Autodesk Inventor part; units mm, degrees
ref_plane "YZ Plane" through (0, 0, 0) normal (1, 0, 0) x (0, 1, 0)
ref_plane "XZ Plane" through (0, 0, 0) normal (0, 1, 0) x (-1, 0, 0)
ref_plane "XY Plane" through (0, 0, 0) normal (0, 0, 1) x (1, 0, 0)
sketch "스케치1" plane through (0, 0, 0) normal (0, 0, 1) x (1, 0, 0)
  line L0 (0, 0) -> (0, 30)
  line L1 (0, 30) -> (1.5, 30)
  line L2 (1.5, 30) -> (1.5, 0)
  line L3 (0, -2) -> (3.5, -2)
  line L4 (3.5, -2) -> (1.5, 0)
  line L5 (0, 0) -> (0, -2)
  dimension "d0" = 30
  dimension "d1" = 7
  dimension "d2" = 3
  dimension "d3" = 45
revolve "회전1" add sketch "스케치1" angle 360 about axis through (0, 0, 0) along (0, 1, 0)
chamfer "모따기1" distance 0.3 angle 45 1 edges at (-1.5, 30, 0)
thread "스레드1"
sketch "스케치2" plane through (0, -2, 0) normal (0, -1, 0) x (1, 0, 0)
  line L0 (-0.5, 2.5) -> (0.5, 2.5)
  line L1 (0.5, 2.5) -> (0.5, -2.5)
  line L2 (0.5, -2.5) -> (-0.5, -2.5)
  line L3 (-0.5, -2.5) -> (-0.5, 2.5)
  circle A0 centre (0, 0) radius 1.2 construction
  line L4 (-0.5, 2.5) -> (0.5, -2.5) construction
  line L5 (0.5, 2.5) -> (-0.5, -2.5) construction
  line L6 (-2.5, -0.5) -> (2.5, -0.5)
  line L7 (2.5, -0.5) -> (2.5, 0.5)
  line L8 (2.5, 0.5) -> (-2.5, 0.5)
  line L9 (-2.5, 0.5) -> (-2.5, -0.5)
  line L10 (-2.5, -0.5) -> (2.5, 0.5) construction
  line L11 (2.5, -0.5) -> (-2.5, 0.5) construction
  point P0 (-0.5, 0.5)
  point P1 (-0.5, -0.5)
  point P2 (0.5, -0.5)
  point P3 (0.5, 0.5)
  dimension "d10" = 1
  dimension "d11" = 5
  dimension "d12" = 5
  dimension "d13" = 1
extrude "돌출1" cut sketch "스케치2" against normal blind 0.5
properties part number "M3 30mm 십자나사"
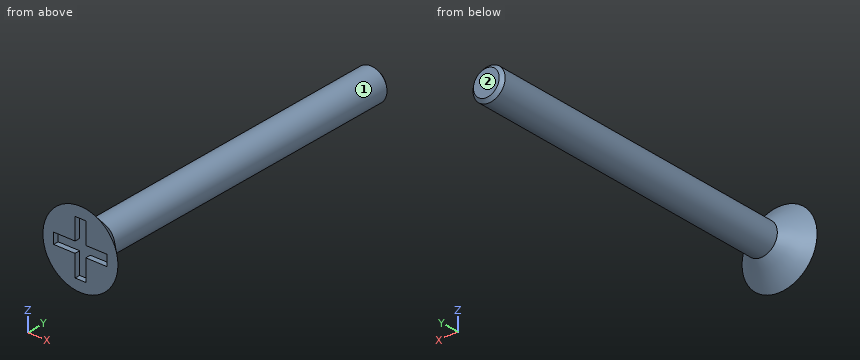
Geometry: final body of the model. Coordinates: model frame, mm. Face numbers are marked on the shaded views. A direction names the side the tool comes from. Give positions to 0.01 mm unless a question says otherwise; leave off trailing zeros. Order: outer loops, then holes, each group sorted by start corner. A loop starts at its lowest first (then second) coordinate and runs counter-clockwise, first axis right, second up. Notation, with made-up numbers: (56.5, 51.5) -> (92.5, 51.5) arc R25 ccw to (92.5, 85.5) -> close; hole circle Ø11 at (47.25, 32). An arc over 180 degrees is marked (long way). Write each question's results on one line, items separated by ' | '.
1) First-contact query: pin 1 Ø4 at (y, z) = (23.5, -1) entering from +X; pin 2 Ø2 at (x, y) = (-1.5, 8) entering from +Z; pin 3 Ø0.6 at (y, z) = (-2, -1) entering from -X. Flat tips, straight axial feed; report the tip coordinate or a pass-through.
Geometry says:
pin 1: stops at x = 1.5 | pin 2: stops at z = 1.41 | pin 3: stops at x = -3.43
2) Line query: line 1 along Z through (x, y) = (-0.5, 14); line 2 along Z through (x, y) = (-1.25, 8); line 3 along Y through (x, z) = (-1.25, -3). Output: solid intervals per line, ascending.
Geometry says:
line 1: z = -1.41 to 1.41 | line 2: z = -0.83 to 0.83 | line 3: y = -2 to -1.75
3) Cut plane A-A (z = 0). Output: boundary loops of the cut face in (x, y), and give its area (3 significant figures).
Geometry says:
outline: (-3.5, -2) -> (-2.5, -2) -> (-2.5, -1.5) -> (2.5, -1.5) -> (2.5, -2) -> (3.5, -2) -> (1.5, 0) -> (1.5, 29.7) -> (1.2, 30) -> (-1.2, 30) -> (-1.5, 29.7) -> (-1.5, 0) -> close | area: 97.4 mm²
4) Set-up query: the marked faces 1 and 2. Return all of +Z, -Z, +X, -X, +Y, -Y with unobstructed straight access to the full face (end or side cutting, diameter ignored); none if empty.
Geometry says:
face 1: +Y | face 2: +Z, -Z, +X, -X, +Y
5) Cut plane C-C (y = 28). Output: boundary loops of the cut face in (x, z).
Geometry says:
outline: circle Ø3 at (0, 0)
6) Cut plane B-B (x = 0). Output: boundary loops of the cut face in (y, z).
Geometry says:
outline: (-2, -3.5) -> (0, -1.5) -> (29.7, -1.5) -> (30, -1.2) -> (30, 1.2) -> (29.7, 1.5) -> (0, 1.5) -> (-2, 3.5) -> (-2, 2.5) -> (-1.5, 2.5) -> (-1.5, -2.5) -> (-2, -2.5) -> close
